```python
from build123d import *


# Not quite as in the source:
# - ends of sketch curves that miss each other by under 0.0002 mm in the source are joined
# - the dataset's text gives a spline's control points without its knots; the knots are read off the source's solid


with BuildPart() as f1:
    # F0 (on Front) → F1 (revolve)
    with BuildSketch(Plane.XZ):
        with BuildLine():
            ThreePointArc((95, 0), (105.6066017178, 4.3933982822), (110, 15))
            Line((110, 15), (110, 52.530664077))
            ThreePointArc((110, 52.530664077), (110.6656938493, 54.229287327), (112.3082567563, 55.0233001372))
            add(Edge.make_bspline(
                [(112.3082567563, 55.0233001372), (112.3371382541, 55.0255218154), (112.3662455353, 55.0279709343), (112.3956622966, 55.030664077)],
                knots=[0.3810790212, 0.3810790212, 0.3810790212, 0.3810790212, 0.3991629595, 0.3991629595, 0.3991629595, 0.3991629595], degree=3))
            add(Edge.make_bspline(
                [(112.3956622966, 55.030664077), (113.3730312437, 55.1201434726), (114.6920333455, 55.4789992419), (114.9571856025, 59.8162261419)],
                knots=[0.3991629595, 0.3991629595, 0.3991629595, 0.3991629595, 1, 1, 1, 1], degree=3))
            ThreePointArc((114.9571856025, 59.8162261419), (114.4670860694, 59.9975450862), (113.9589484435, 59.8756013901))
            add(Edge.make_bspline(
                [(112.3044930104, 56.0264915082), (112.3140793136, 56.0273704068), (112.3650984167, 56.0322078345), (112.4927350046, 56.0466584989), (112.6564819563, 56.0784065116), (112.8095723323, 56.1345234503), (112.9464281063, 56.217405399), (113.1051907024, 56.367326932), (113.2969685197, 56.6463774626), (113.5030707113, 57.1049132693), (113.7625500872, 57.9971767083), (113.9062854104, 59.0152971487), (113.9589484435, 59.8756013901)],
                knots=[0.3990705563, 0.3990705563, 0.3990705563, 0.3990705563, 0.40625, 0.4375, 0.5, 0.5625, 0.625, 0.6875, 0.75, 0.8125, 0.875, 0.9999203957, 0.9999203957, 0.9999203957, 0.9999203957], degree=3))
            Line((112.3044930104, 56.0264915082), (108.406190974, 56.0264994193))
            ThreePointArc((108.406190974, 56.0264994193), (106.8803038189, 55.787976962), (105.5000000054, 55.0951667753))
            Line((105.5000000054, 55.0951667753), (105.5, 15))
            ThreePointArc((105.5, 15), (102.4246212025, 7.5753787975), (95, 4.5))
            Line((95, 4.5), (92.4233198166, 4.5))
            Line((92.4233198166, 4.5), (0, 4.5))
            Line((0, 4.5), (0, 0))
            Line((0, 0), (92.4233198166, 0))
            Line((92.4233198166, 0), (95, 0))
        make_face()
        with BuildLine():
            add(Edge.make_bspline(
                [(112.3082567563, 55.0233001372), (112.3371382541, 55.0255218154), (112.3662455353, 55.0279709343), (112.3956622966, 55.030664077)],
                knots=[0.3810790212, 0.3810790212, 0.3810790212, 0.3810790212, 0.3991629595, 0.3991629595, 0.3991629595, 0.3991629595], degree=3))
            ThreePointArc((112.3082567563, 55.0233001372), (112.4040577008, 55.0288224137), (112.5, 55.030664077))
            Line((112.5, 55.030664077), (112.3956622966, 55.030664077))
        make_face()
    revolve(axis=Axis((0, 0, 2.25), (0, 0, 1)))


solid = f1.part
```
The model under review builds one solid part; all positions refer to its coordinate system, in mm. Give positions to 0.01 mm unless a question says otherwise; leave off trailing zeros. Write each loop counter-clockwise with the first axis right and the second up, starting at its lowest first coordinate (ties: lowest second). Pieces come first, ordered by that corner, then holes. Notation, with made-up numbers: (58.5, -22) - (89.5, -22) arc R12 ccw to (89.5, -17) - close; hole circle Ø9 at (-31.5, 55.5). An arc over 180 degrees is marked (long way). Answer in a Markdown table with one row per item. Add a question column.
1. Wall thickness on line 1 along Y through (x, z) = (0, 45); line 2 along Y through (x, z) = (3, 38); line 3 along X through (y, z) = (-87.5, 50): over which ranges is each line inside the solid? List them lowest first. Write a range as [from, to].
2. Insertion check: P1, Ø1, axis at x = -18, z = 18.5, coming from the +Y side; P2, Ø8, axis at y = -77, z = 31.5, coming from the +X side; P3, Ø3, axis at x = 4, z = 14.5, coming from the +Y side. Each pin has a flat end and moves straight along its axis. Give the tip position at first contact, or say it passes through.
3. We need section B-B on z = 10.5. Write out the cut boundary in (x, y).
4. We need section A-A on z = 45. Write out the cut boundary in (x, y).
5. Draft analysis for pull direction Y (two halves, no side actions). For faces 1 (the conical face through (-86.178, -66.079, 56.026)), 2 (the flat face through (1, 1, 0)), 3 (the cylindrical face through (-23.846, -107.384, 34.028)), state which applies: +Y half, -Y half, draft (parallel to the pull), parting line (faces both ways), or undercut.
Ans:
| question | item | result |
|---|---|---|
| 1 | line 1 | y = [-110, -105.5], [105.5, 110] |
| 1 | line 2 | y = [-109.96, -105.46], [105.46, 109.96] |
| 1 | line 3 | x = [-66.66, -58.94], [58.94, 66.66] |
| 2 | P1 | stops at y = 108.6 |
| 2 | P2 | stops at x = 82.29 |
| 2 | P3 | stops at y = 109.97 |
| 3 | outline | circle Ø218.62 at (0, 0); hole circle Ø208.97 at (0, 0) |
| 4 | outline | circle Ø220 at (0, 0); hole circle Ø211 at (0, 0) |
| 5 | face 1 | undercut |
| 5 | face 2 | draft |
| 5 | face 3 | parting line |
